Part model, mm, in its own coordinate system. A direction names the side the tool comes from. Round coordinates to 2 decimals unless told otherwise and drop trailing zeros. Loops run counter-clockwise (first coordinate to the right, second up) from the corner with the lowest first, then second, coordinate; pieces in that order, holes last.
(1) Tool access for faces 1 (the face through (3.208, 14.79, -14.448)), 2 (the face through (-7.4, -6, -12.1)): list every direction of +Z, -Z, +X, -X, +Y, -Y with a clear straight run to the whole face (end or side of a thin tool).
(2) Mould opens along X. For faces 3 (the face through (-9, 30, -10)), 4 (the face through (-13.887, -2.465, -10.648)), 5 (the face through (10.316, 12.745, -7.91)) say: +X half, -X half, draft (parallel to the pull), parting line (faces both ways), or undercut.
(3) Cut at B-B on x = 0. List the corners of the cut face in (y, z).
(4) Flat gauge pins, fed straight in: pin 1 (2 mm diameter, centred on y = 25.5, z = -7, fed in from +X); pin 2 (4 mm diameter, centred on x = -12, y = 17, fed in from -Z); pin 3 (1 mm diameter, centred on y = 8, z = -2, fed in from -X). Where does each tip first touch, or does it go through?
(5) Cut at C-C on y = 21. List the corners of the cut face in (x, z).
(6) Cut at A-A on z = 0. List the corners of the cut face in (x, y).
(7) Probe probe 1 along Z at (x, y) = (0, 20.5); probe 2 along X at (y, z) = (9.5, 6); probe 3 along Y at (x, z) = (0.5, -15). List the from-to ranges inside material, lowest first.
from build123d import *

# Parameters (mm, degrees)
F0_R           = 17.5
F1_DEPTH       = 6
F2_R           = 1
F3_R           = 14.8
F4_DEPTH       = 30
F6_D           = 26
F6_DEPTH       = 60
F6_CSINK_D     = 28
F6_CSINK_ANGLE = 90


with BuildPart() as f1:
    # F0 (on Front) → F1 (new body)
    with BuildSketch(Plane.XZ):
        Circle(F0_R)
    extrude(amount=F1_DEPTH)

    # F2
    f2_edges = [f1.edges().sort_by_distance(p)[0] for p in [
        (-17.5, -6, 0),
    ]]
    fillet(f2_edges, radius=F2_R)

    # F3 (on face) → F4 (join)
    with BuildSketch(Plane(origin=(0, 0, 0), x_dir=(-1, 0, 0), z_dir=(0, 1, 0))):
        Circle(F3_R)
    extrude(amount=F4_DEPTH)

    # F6
    with Locations(Plane.XZ.offset(6)):
        with Locations((0, 0)):
            CounterSinkHole(F6_D / 2, F6_CSINK_D / 2, depth=F6_DEPTH, counter_sink_angle=F6_CSINK_ANGLE)


solid = f1.part
Final values:
1. face 1: +Y
1. face 2: +Z, -Z, +X, -X, -Y
2. face 3: draft
2. face 4: parting line
2. face 5: undercut
3. outline: (-6, -16.5) arc R1 ccw to (-5, -17.5) - (0, -17.5) - (0, -14.8) - (30, -14.8) - (30, -13) - (-5, -13) - (-6, -14) - close; (-6, 14) - (-5, 13) - (30, 13) - (30, 14.8) - (0, 14.8) - (0, 17.5) - (-5, 17.5) arc R1 ccw to (-6, 16.5) - close
4. pin 1: stops at x = 13.53
4. pin 2: stops at z = -10.91
4. pin 3: stops at x = -14.72
5. outline: circle Ø29.6 at (0, 0); hole circle Ø26 at (0, 0)
6. outline: (-17.5, -5) arc R1 ccw to (-16.5, -6) - (-14, -6) - (-13, -5) - (-13, 30) - (-14.8, 30) - (-14.8, 0) - (-17.5, 0) - close; (13, -5) - (14, -6) - (16.5, -6) arc R1 ccw to (17.5, -5) - (17.5, 0) - (14.8, 0) - (14.8, 30) - (13, 30) - close
7. probe 1: z = -14.8 to -13, 13 to 14.8
7. probe 2: x = -13.53 to -11.53, 11.53 to 13.53
7. probe 3: y = -6 to 0
